Source: CAD feature listing. Evaluate the final solid. Frame: model axes, mm. A direction names the side the tool comes from. Coordinates: 2 decimals unless noted, no trailing zeros. Write each loop counter-clockwise with the first axis right and the second up, starting at its lowest first coordinate (ties: lowest second). Pieces come first, ordered by that corner, then holes. Notation, with made-up numbers: M -35,69 L -21,69 A28 cw -21,88 Z; hole C 63.25,53.25 d9. An arc over 180 degrees is marked long. Answer as CSV lines item,"result". Start each with the question number.
1. Section D-D on z = -231.5. Return the cut outline in (x, y).
2. Contact query for flat-ended pins moving along their axis: pin 1 Ø6 at (y, z) = (-63.5, 223) entering from -X; pin 2 Ø6 at (x, z) = (54.5, 225) entering from -Y; pin 3 Ø1 at (x, z) = (-79.5, -239.5) entering from +Y. Output: stop coordinate, or through.
3. Section A-A on y = 0. Return the cut outline in (x, z), plus the area to 3 significant figures.
4. Mould query, pull axis Y, two halves, no side actions, for faces 1 (the face through (2, -125, 0)), 2 (the face through (1.4, 297.447, 39.054)), 3 (the face through (150, -31, -98)). Classes: pulls with the +Y half, pulls with the -Y half, needs draft (parallel to the pull), parting line crosses it, or undercut.
5. Section B-B on z = -35. Return the cut outline in (x, y), plus the area to 3 significant figures.
6. Section C-C on x = -108. Return the cut outline in (y, z), plus the area to 3 significant figures.
7. Reachability of faces 4 (the face through (100, -243, -132)), 5 (the face through (-40, -118, -118)), 6 (the face through (2, -111, -25)) from +Z, -Z, +X, -X, +Y, -Y: full face, straight path, thin tool, end or side. Return the list, or none.
8. Line query: probe 1 along Y at (x, z) = (71, 0); probe 2 along Y at (x, z) = (-136.5, -5.5); probe 3 along Z at (x, y) = (-77.5, -55). Output: solid intervals per line, ascending. Write a range as [from, to].
```python
from build123d import *

# Parameters (mm, degrees)
IZIM1_R                     = 150
Y_KSEKLIK_EKSTR_ZYON1_DEPTH = 150
IZIM2_R                     = 300
IZIM2_R_2                   = 275
Y_KSEKLIK_EKSTR_ZYON2_DEPTH = 100
IZIM3_R                     = 275
IZIM3_R_2                   = 150
Y_KSEKLIK_EKSTR_ZYON3_DEPTH = 40


with BuildPart() as part:
    # izim1 → Y_kseklik-Ekstr_zyon1 (new, symmetric)
    with BuildSketch(Plane(origin=(0, 0, 0), x_dir=(0, 0, -1), z_dir=(1, 0, 0))):
        Circle(IZIM1_R)
        with BuildLine():
            Line((-25, -125), (25, -125))
            Line((25, -125), (25, -96.824583655))
            ThreePointArc((25, -96.824583655), (0, 100), (-25, -96.824583655))
            Line((-25, -96.824583655), (-25, -125))
        make_face(mode=Mode.SUBTRACT)
    extrude(amount=Y_KSEKLIK_EKSTR_ZYON1_DEPTH, both=True)



with BuildPart() as body_2:
    # izim2 → Y_kseklik-Ekstr_zyon2 (new, symmetric)
    with BuildSketch(Plane(origin=(0, 0, 0), x_dir=(0, 0, -1), z_dir=(1, 0, 0))):
        Circle(IZIM2_R)
        Circle(IZIM2_R_2, mode=Mode.SUBTRACT)
    extrude(amount=Y_KSEKLIK_EKSTR_ZYON2_DEPTH, both=True)


with BuildPart() as part_1:
    add(part.part)

    add(body_2.part)  # Y_kseklik-Ekstr_zyon3 merges body 2
    # izim3 → Y_kseklik-Ekstr_zyon3 (add, symmetric)
    with BuildSketch(Plane(origin=(0, 0, 0), x_dir=(0, 0, -1), z_dir=(1, 0, 0))):
        Circle(IZIM3_R)
        Circle(IZIM3_R_2, mode=Mode.SUBTRACT)
    extrude(amount=Y_KSEKLIK_EKSTR_ZYON3_DEPTH, both=True)


solid = part_1.part
```
Values:
1,outline,"M -100,-190.81 L 100,-190.81 L 100,-148.43 L 40,-148.43 L 40,148.43 L 100,148.43 L 100,190.81 L -100,190.81 L -100,148.43 L -40,148.43 L -40,-148.43 L -100,-148.43 Z"
2,pin 1,"x = -40"
2,pin 2,"y = -201.78"
2,pin 3,"y = 181.33"
3,outline,"M -150,-150 L -40,-150 L -40,-275 L -100,-275 L -100,-300 L 100,-300 L 100,-275 L 40,-275 L 40,-150 L 150,-150 L 150,-100 L -150,-100 Z; M -150,100 L 150,100 L 150,150 L 40,150 L 40,275 L 100,275 L 100,300 L -100,300 L -100,275 L -40,275 L -40,150 L -150,150 Z"
3,area,"60,000 mm²"
4,face 1,"undercut"
4,face 2,"parting line crosses it"
4,face 3,"needs draft"
5,outline,"M -150,-145.86 L -40,-145.86 L -40,-272.76 L -100,-272.76 L -100,-297.95 L 100,-297.95 L 100,-272.76 L 40,-272.76 L 40,-145.86 L 150,-145.86 L 150,-93.67 L -150,-93.67 Z; M -150,93.67 L 150,93.67 L 150,145.86 L 40,145.86 L 40,272.76 L 100,272.76 L 100,297.95 L -100,297.95 L -100,272.76 L -40,272.76 L -40,145.86 L -150,145.86 Z"
5,area,"61,700 mm²"
6,outline,"C 0,0 d300; hole M -125,-25 L -96.82,-25 A100 ccw long -96.82,25 L -125,25 Z"
6,area,"38,000 mm²"
7,face 4,"+X"
7,face 5,"-X"
7,face 6,"+X, -X"
8,probe 1,"[-300, -275], [-150, -125], [100, 150], [275, 300]"
8,probe 2,"[-149.9, -125], [99.85, 149.9]"
8,probe 3,"[-294.92, -269.44], [-139.55, -83.52], [83.52, 139.55], [269.44, 294.92]"
